from build123d import *

# Parameters (mm, degrees)
F0_W     = 140
F0_H     = 60
F1_DEPTH = 60
F3_R     = 10
F5_DEPTH = 10
F4_R     = 10
F6_DEPTH = 73.6


with BuildPart() as f1:
    # F0 (on Top) → F1 (new body)
    with BuildSketch(Plane.XY):
        Rectangle(F0_W, F0_H)
    extrude(amount=F1_DEPTH)

    # F3 (on face) → F5 (join)
    with BuildSketch(Plane.XY.offset(60)):
        with Locations((-30.702168, 0.617491)):
            Circle(F3_R)
    extrude(amount=F5_DEPTH)

    # F4 (on face) → F6 (cut)
    with BuildSketch(Plane.XY.offset(60)):
        Circle(F4_R)
    extrude(amount=-F6_DEPTH, mode=Mode.SUBTRACT)


solid = f1.part
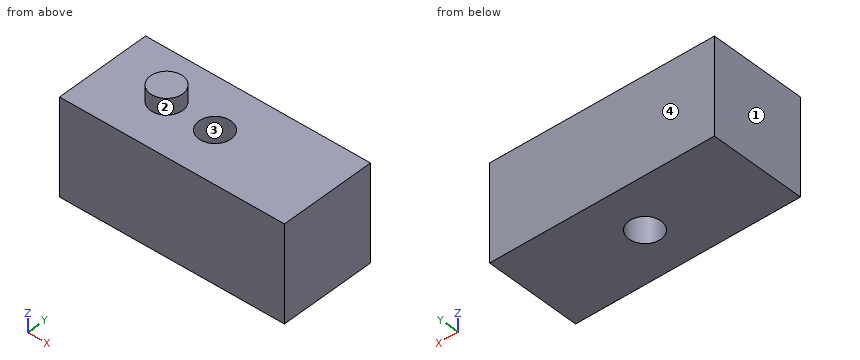
Could you check a few things on this model? Use its own coordinates, in mm. Face numbers are marked on the shaded views. Round coordinates to 2 decimals unless told otherwise and drop trailing zeros. Order: outer loops, then holes, each group sorted by start corner. A loop starts at its lowest first (then second) coordinate and runs counter-clockwise, first axis right, second up.
Q1. Imagine slicing it at B-B, the plane z = 43.5. List the corners of the cut face in (x, y) for me, then the cut area to 3 significant figures.
Geometry says:
outline: (-70, -30) - (70, -30) - (70, 30) - (-70, 30) - close; hole circle Ø20 at (0, 0)
area: 8,090 mm2
Q2. Imagine slicing it at A-A, the plane x = 0. List the corners of the cut face in (y, z) for me.
Geometry says:
outline: (-30, 0) - (-10, 0) - (-10, 60) - (-30, 60) - close; (10, 0) - (30, 0) - (30, 60) - (10, 60) - close
Q3. Thinking about a two-plate mould opening in X: for the marked faces 1, 2, 3 and 4, which applies, released by +X, released by -X, zero draft, split by the parting line, or undercut?
Geometry says:
face 1: released by -X
face 2: split by the parting line
face 3: undercut
face 4: zero draft
Q4. Imagine slicing it at C-C, the plane x = -32.5. List the corners of the cut face in (y, z) for me.
Geometry says:
outline: (-30, 0) - (30, 0) - (30, 60) - (10.45, 60) - (10.45, 70) - (-9.22, 70) - (-9.22, 60) - (-30, 60) - close
Q5. I'm going to push flat-ended pins straight in: P1, Ø1.5, axis at x = -2, y = 7, coming from the +Z side; P2, Ø1, axis at y = 4, z = 62.5, coming from the -X side; P3, Ø3, axis at x = 24.5, y = -20, coming from the +Z side. Where does each tip first touch, or does it pass through?
Geometry says:
P1: passes through
P2: stops at x = -40.28
P3: stops at z = 60
Q6. Please list where these lines run through material, in increasing order: probe 1 along Y at (x, z) = (0, 47); probe 2 along Z at (x, y) = (-32, -16.5); probe 3 along X at (y, z) = (8, 41.5).
Geometry says:
probe 1: y = -30 to -10, 10 to 30
probe 2: z = 0 to 60
probe 3: x = -70 to -6, 6 to 70
